Print and shaded views of the part. All mm, measured from the part's lowest x, y and z. A direction names the side the tool comes from. Round coordinates to 2 decimals unless told otherwise and drop trailing zeros. Order: outer loops, then holes, each group sorted by start corner. A loop starts at its lowest first (then second) coordinate and runs counter-clockwise, first axis right, second up. Notation, with made-up numbers: (46, 67) - (91, 67) arc R16 ccw to (91, 88) - close; hole circle Ø5 at (31.5, 87.25). An arc over 180 degrees is marked (long way). Write item = value, one per line.
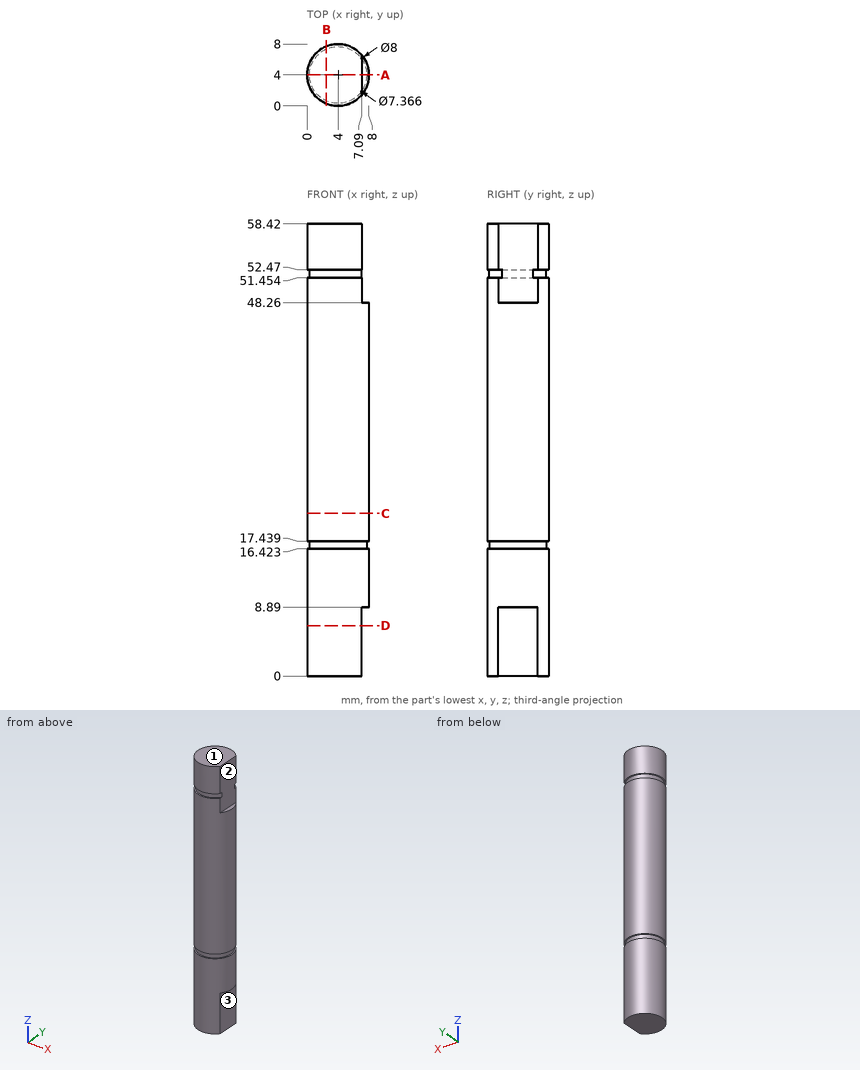
(1) Tool access for the marked faces 1, 2 and 3: list every direction of +Z, -Z, +X, -X, +Y, -Y with a clear straight run to the whole face (end or side of a thin tool).
Solved:
face_1 = +Z, +X, -X, +Y, -Y
face_2 = +Z, +X, +Y, -Y
face_3 = -Z, +X, +Y, -Y
(2) Band-saw the part on C-C on z = 21. List the corners of the cut face in (x, y).
Solved:
outline = circle Ø8 at (4, 4)
(3) Probe line 1 along Y through (x, z) = (3.75, 39); line 2 along X through (y, z) = (5, 53). List the from-to ranges inside material, lowest first.
Solved:
line_1 = 0.01 to 7.99
line_2 = 0.13 to 7.09
(4) Drop flat-ended pins along their axis: pin 1 (1 mm diameter, centred on x = 7, z = 48.5, fed in from +Y); pin 2 (2 mm diameter, centred on x = 3.5, y = 4, fed in from -Z); pin 3 (2 mm diameter, centred on x = 1, z = 10.5, fed in from +Y) (1 decimal); pin 4 (1.5 mm diameter, centred on y = 3.5, z = 6, fed in from +X). Give the stop position or say it passes through.
Solved:
pin_1 = 7.12
pin_2 = 0
pin_3 = 7.5
pin_4 = 7.09
(5) Band-saw the part on A-A on y = 4. List the corners of the cut face in (x, z).
Solved:
outline = (0, 0) - (7.09, 0) - (7.09, 8.89) - (8, 8.89) - (8, 16.42) - (7.68, 16.42) - (7.68, 17.44) - (8, 17.44) - (8, 48.26) - (7.09, 48.26) - (7.09, 58.42) - (0, 58.42) - (0, 52.47) - (0.32, 52.47) - (0.32, 51.45) - (0, 51.45) - (0, 17.44) - (0.32, 17.44) - (0.32, 16.42) - (0, 16.42) - close
(6) Band-saw the part on B-B on x = 2.5. List the corners of the cut face in (y, z), plus the area to 3 significant figures.
Solved:
outline = (0.29, 0) - (7.71, 0) - (7.71, 16.42) - (7.36, 16.42) - (7.36, 17.44) - (7.71, 17.44) - (7.71, 51.45) - (7.36, 51.45) - (7.36, 52.47) - (7.71, 52.47) - (7.71, 58.42) - (0.29, 58.42) - (0.29, 52.47) - (0.64, 52.47) - (0.64, 51.45) - (0.29, 51.45) - (0.29, 17.44) - (0.64, 17.44) - (0.64, 16.42) - (0.29, 16.42) - close
area = 432 mm²
(7) Band-saw the part on D-D on z = 6.5. List the corners of the cut face in (x, y).
Solved:
outline = (7.09, 1.46) - (7.09, 6.54) arc R4 ccw (long way) to start
